Part model, mm, in its own coordinate system. A direction names the side the tool comes from. Coordinates: 2 decimals unless noted, no trailing zeros. Order: outer loops, then holes, each group sorted by start corner. A loop starts at its lowest first (then second) coordinate and runs counter-clockwise, first axis right, second up.
1) Pin check, flat tips, straight feed: pin 1 Ø1 at (x, y) = (-17.5, -5.5) entering from +Z; pin 2 Ø7 at (x, y) = (-29, -36.5) entering from -Z; pin 3 Ø5 at (y, z) = (24, 7.5) entering from -X; pin 4 Ø3.5 at (x, y) = (-29, 36.5) entering from -Z. Stop position of each tip, or through.
2) Cut at B-B (y = 2.5). List the corners of the cut face in (x, z), and give its area (3 significant figures).
3) Mould opens along X. For faces 1 (the flat face through (29.87, 32.45, 9.61)), 2 (the flat face through (-28, -35, 15)), 3 (the flat face through (25, 3.5, 11)), 4 (the flat face through (-35, 1, 1)) say: +X half, -X half, draft (parallel to the pull), parting line (faces both ways), or undercut.
4) Wall check: L1, parallel to Y at x = 20, z = 16.75; L2, parallel to X at y = -36.5, z = 16.45; L3, parallel to Y at x = -29, z = 1.25. Give the ranges that are in metal, low to high.
5) Tool access for faces 5 (the cylindrical face through (26.79, -38.53, 7.4)), 6 (the flat face through (29.757, 18.385, 5.28)), 7 (the cylindrical face through (17, 9.6, 14.5)), 8 (the flat face through (-24.31, -40.907, 10.872)): list every direction of +Z, -Z, +X, -X, +Y, -Y with a clear straight run to the whole face (end or side of a thin tool).
6) Cut at A-A (x = 6.5). List the corners of the cut face in (y, z), and give its area (3 significant figures).
7) Cut at C-C (z = 12.5). Give the number of separate pieces and of enclosed holes in the cut face, and give its area (3 significant figures).
```python
from build123d import *

# Parameters (mm, degrees)
SKETCH002_R     = 1.6
PAD001_DEPTH    = 19.5
POCKET001_DEPTH = 17.5
SKETCH005_R     = 3
POCKET002_DEPTH = 15
SKETCH006_R     = 3
POCKET003_DEPTH = 3.5
POCKET004_DEPTH = 2
SKETCH008_W     = 14
SKETCH008_H     = 9
POCKET005_DEPTH = 2


with BuildPart() as part:
    # Sketch002 → Pad001 (new body)
    with BuildSketch(Plane.XY):
        with BuildLine():
            Line((-35, 36.5000000001), (-35, -36.5))
            ThreePointArc((-35, -36.5), (-33.2426406871, -40.7426406871), (-29, -42.5))
            Line((-29, -42.5), (29, -42.5))
            ThreePointArc((29, -42.5), (33.2426406868, -40.7426406875), (35, -36.500000001))
            Line((35, -36.500000001), (35.0000000077, 8.799999999))
            ThreePointArc((35.0000000077, 8.799999999), (34.9358203402, 9.2874929726), (34.747655076, 9.7417641056))
            Line((24.9046932533, 26.7902740862), (34.747655076, 9.7417641056))
            ThreePointArc((25.7902740862, 30.0953067467), (24.6629889937, 28.6262002123), (24.9046932533, 26.7902740862))
            Line((25.7902740862, 30.0953067467), (34.0582358931, 34.8688167197))
            ThreePointArc((34.0582358931, 34.8688167197), (34.7476550681, 35.5582358947), (34.9999999999, 36.5000000017))
            ThreePointArc((34.9999999999, 36.5000000017), (33.2426406864, 40.7426406877), (28.9999999999, 42.5))
            Line((28.9999999999, 42.5), (-29.0000000001, 42.5))
            ThreePointArc((-29.0000000001, 42.5), (-33.2426406871, 40.7426406871), (-35, 36.5000000001))
        make_face()
        with Locations((28.9999999999, 36.5)):
            Circle(SKETCH002_R, mode=Mode.SUBTRACT)
        with Locations((29, -36.5)):
            Circle(SKETCH002_R, mode=Mode.SUBTRACT)
        with Locations((-29, -36.5)):
            Circle(SKETCH002_R, mode=Mode.SUBTRACT)
        with Locations((-29.0000000001, 36.5000000001)):
            Circle(SKETCH002_R, mode=Mode.SUBTRACT)
    extrude(amount=PAD001_DEPTH)

    # Sketch003 (on Face19 of Pad001) → Pocket001 (cut)
    with BuildSketch(Plane.XY.offset(19.5)):
        with BuildLine():
            ThreePointArc((25.2287638336, 37.8333333333), (25.0151381406, 36.1523277954), (25.516649593, 34.5337167186))
            ThreePointArc((24.7749743893, 31.8185242701), (25.7042911697, 33.0235677135), (25.516649593, 34.5337167186))
            ThreePointArc((24.7749743893, 31.8185242701), (22.7240689546, 29.1457322713), (23.1638091612, 25.8055737838))
            Line((23.1638091612, 25.8055737838), (32.7320508154, 9.2328930931))
            ThreePointArc((33.0000000077, 8.2328930934), (32.9318516603, 8.7505311835), (32.7320508154, 9.2328930931))
            Line((33.0000000077, 8.2328930934), (33.0000000077, 3.5))
            Line((18.0000000077, 3.5), (33.0000000077, 3.5))
            Line((18.0000000077, 40.5), (18.0000000077, 3.5))
            Line((23.3431457504, 40.5), (18.0000000077, 40.5))
            ThreePointArc((25.2287638336, 37.8333333333), (24.9761389123, 39.6547005384), (23.3431457504, 40.5))
        make_face()
        with BuildLine():
            ThreePointArc((31.4000000061, -33.3000000046), (26.171572878, -33.6715728725), (25.8, -38.9))
            ThreePointArc((25, -40.5), (25.894427191, -39.9472135955), (25.8, -38.9))
            Line((25, -40.5), (-21.8058862217, -40.5))
            ThreePointArc((-21.947307578, -40.4414213562), (-21.8824229082, -40.4847759065), (-21.8058862217, -40.5))
            Line((-21.947307578, -40.4414213562), (-25.0071533734, -37.3815755608))
            ThreePointArc((-25.0626019212, -37.2049087662), (-25.0565540108, -37.3000454956), (-25.0071533734, -37.3815755608))
            ThreePointArc((-25.0626019212, -37.2049087662), (-32.5456214666, -34.648360614), (-26.1715722902, -39.3284265397))
            ThreePointArc((-25.8887295485, -39.3284265105), (-26.0301509254, -39.2698478667), (-26.1715722902, -39.3284265397))
            Line((-22.7757347027, -42.4414213562), (-25.8887295485, -39.3284265105))
            ThreePointArc((-22.7757347027, -42.4414213562), (-22.710850033, -42.4847759065), (-22.6343133465, -42.5))
            Line((-29, -42.5), (-22.6343133465, -42.5))
            ThreePointArc((-35, -36.5), (-33.2426406871, -40.7426406871), (-29, -42.5))
            Line((-35, -36.5), (-35, 36.4999997364))
            ThreePointArc((-35, 36.4999997364), (-27.6821008816, 30.6465273631), (-23.5789525827, 39.0714285714))
            ThreePointArc((-22.6754446798, 40.5), (-23.5205989345, 40.0345224838), (-23.5789525827, 39.0714285714))
            Line((16.0000000077, 40.5), (-22.6754446798, 40.5))
            Line((16.0000000077, 40.5), (16.0000000077, 3.5))
            Line((-32, 3.5), (16.0000000077, 3.5))
            Line((-32, 1.5), (-32, 3.5))
            Line((33.0000000077, 1.5), (-32, 1.5))
            Line((33.0000000077, 1.5), (33.0000000077, -32.5000000058))
            ThreePointArc((31.4000000061, -33.3000000046), (32.4472136023, -33.3944271972), (33.0000000077, -32.5000000058))
        make_face()
    extrude(amount=-POCKET001_DEPTH, mode=Mode.SUBTRACT)

    # Sketch004 (on DatumLine) → Groove (revolve, cut)
    with BuildSketch(Plane(origin=(-29.0000000001, 36.5000000001, 19.5), x_dir=(1, 0, 0), z_dir=(0, -1, 0))):
        Polygon((-5.9999999999, 0), (-5.9999999999, -15.5), (-4.4999999999, -15.5), (-2, 0), align=None)
    revolve(axis=Axis((-29.0000000001, 36.5000000001, 19.5), (0, 0, 1)), mode=Mode.SUBTRACT)

    # Sketch005 (on Face4 of Groove) → Pocket002 (cut)
    with BuildSketch(Plane(origin=(0, 0, 0), x_dir=(1, 0, 0), z_dir=(0, 0, -1))):
        with Locations((29, -36.5)):
            Circle(SKETCH005_R)
        with Locations((29, 36.5)):
            Circle(SKETCH005_R)
        with Locations((-29, 36.5)):
            Circle(SKETCH005_R)
    extrude(amount=-POCKET002_DEPTH, mode=Mode.SUBTRACT)

    # Sketch006 (on Face4 of Pocket002) → Pocket003 (cut)
    with BuildSketch(Plane(origin=(0, 0, 0), x_dir=(1, 0, 0), z_dir=(0, 0, -1))):
        with Locations((-29, -36.5)):
            Circle(SKETCH006_R)
    extrude(amount=-POCKET003_DEPTH, mode=Mode.SUBTRACT)

    # Sketch007 (on Face35 of Pocket003) → Pocket004 (cut)
    with BuildSketch(Plane(origin=(16.0000000077, 0, 0), x_dir=(0, -1, 0), z_dir=(-1, 0, 0))):
        with BuildLine():
            ThreePointArc((-14.5, 19.5), (-9.5, 14.5), (-4.5, 19.5))
            Line((-14.5, 19.5), (-4.5, 19.5))
        make_face()
    extrude(amount=-POCKET004_DEPTH, mode=Mode.SUBTRACT)

    # Sketch008 (on Face6 of Pocket004) → Pocket005 (cut)
    with BuildSketch(Plane(origin=(30.2790489079, 17.4816170309, 0), x_dir=(-0.4999999999, 0.8660254039, 0), z_dir=(0.8660254039, 0.4999999999, 0))):
        with Locations((0.9057494867, 10.75)):
            Rectangle(SKETCH008_W, SKETCH008_H)
    extrude(amount=-POCKET005_DEPTH, mode=Mode.SUBTRACT)


solid = part.part
```
Geometry check:
1. pin 1: stops at z = 2
1. pin 2: stops at z = 0
1. pin 3: stops at x = 16
1. pin 4: stops at z = 3.5
2. outline: (-35, 0) - (35, 0) - (35, 19.5) - (-32, 19.5) - (-32, 2) - (-35, 2) - close
2. area: 1,310 mm2
3. face 1: +X half
3. face 2: undercut
3. face 3: undercut
3. face 4: -X half
4. L1: y = -42.5 to -40.5, 1.5 to 3.5, 40.5 to 42.5
4. L2: x = -33 to -30.6, -27.4 to -25, 25 to 27.4, 30.6 to 35
4. L3: y = -42.5 to -39.5, -33.5 to 33.5, 39.5 to 42.5
5. face 5: -Z
5. face 6: +Z, -Z, +X
5. face 7: +Z, -X
5. face 8: +Z, -Y
6. outline: (-42.5, 0) - (42.5, 0) - (42.5, 19.5) - (40.5, 19.5) - (40.5, 2) - (3.5, 2) - (3.5, 19.5) - (1.5, 19.5) - (1.5, 2) - (-40.5, 2) - (-40.5, 19.5) - (-42.5, 19.5) - close
6. area: 275 mm2
7. separate pieces: 2
7. enclosed holes: 4
7. area: 678 mm2
